Geometry: final body of the model. Coordinates: model frame, mm. A direction names the side the tool comes from. Round coordinates to 2 decimals unless told otherwise and drop trailing zeros. Write each loop counter-clockwise with the first axis right and the second up, starting at its lowest first coordinate (ties: lowest second). Pieces come first, ordered by that corner, then holes. Notation, with made-up numbers: M 33.5,-32 L 83.5,-32 A27 cw 83.5,-12 Z; hole C -1,85 d2. An arc over 180 degrees is marked long. Use one line per item in the form item = value. Start each with the question number.
Item 1: Section query C-C (z = 488.5). Return loops of the section in (x, y), and give its area (3 significant figures).
Item 2: Section query B-B (y = 23). Return loops of the section in (x, z), and give its area (3 significant figures).
Item 3: Pull-direction query (Y, two-part tool) for faces 6 (the flat face through (-216, -876.829, 392)), 7 (the flat face through (-216, 68.051, 807)), 8 (the flat face through (-216, -142, 731.52)), 9 (the flat face through (18.22, 418.85, 450.8)); classes: pulls with the +Y half, pulls with the -Y half, needs draft (parallel to the pull), parting line crosses it, or undercut.
Item 4: Ray query, probe 1 along X at (y, z) = (-590, 610); probe 2 along Y at (x, z) = (31.5, 634.5); probe 3 along X at (y, z) = (-269, 721.5). Return the intervals inside material, ascending.
Item 5: Section query A-A (z = 141). Return loops of the section in (x, y).
Item 6: Pin query (flat end, axial travel): pin 1 Ø15 at (x, z) = (-250.5, 463.5) entering from +Y; pin 2 Ø1.5 at (y, z) = (192, 397.5) entering from -X; pin 3 Ø24.5 at (x, z) = (-218.5, 789) entering from -Y; pin 4 Ø5 at (x, y) = (-175.5, -206) entering from -Z. Return the tip coordinate at first contact, or that it passes through.
Item 7: Section query D-D (x = 8). Return loops of the section in (y, z).
Item 8: Reachability of faces 1 (the flat face through (-216, -450.109, 392)), 2 (the flat face through (-216, -660, 883.92)), 3 (the flat face through (10, -307, 914.4)), 4 (the flat face through (-216, -142, 91.44)), 5 (the flat face through (-216, -876.829, 807)) from +Z, -Z, +X, -X, +Y, -Y: full face, straight path, thin tool, end or side. Return the list, or none.
from build123d import *

# Parameters (mm, degrees)
F1_DEPTH = 914.4
F2_W     = 426.72
F2_H     = 609.6
F2_H_2   = 152.4
F3_DEPTH = 30.48
F4_W     = 15.24
F4_H     = 121.92
F5_DEPTH = 30.48


with BuildPart() as f1:
    # F0 (on Top) → F1 (new body)
    with BuildSketch(Plane.XY):
        Polygon((318.431516, 193.019261), (-290.511489, 651.093946), (-280.741865, 224.485797), (-201.23198, 132.059261), (-201.23198, -934.740739), (318.431516, -934.740739), align=None)
    extrude(amount=F1_DEPTH)

    # F2 (on face) → F3 (join)
    with BuildSketch(Plane(origin=(-201.23198, 0, 0), x_dir=(0, -1, 0), z_dir=(-1, 0, 0))):
        with Locations((145.308739, 396.24)):
            Rectangle(F2_W, F2_H)
        with Locations((663.468739, 396.24)):
            Rectangle(F2_W, F2_H)
        with Locations((145.308739, 807.72)):
            Rectangle(F2_W, F2_H_2)
        with Locations((663.468739, 807.72)):
            Rectangle(F2_W, F2_H_2)
    extrude(amount=F3_DEPTH)

    # F4 (on face) → F5 (join)
    with BuildSketch(Plane(origin=(-231.71198, 0, 0), x_dir=(0, -1, 0), z_dir=(-1, 0, 0))):
        with Locations((329.712739, 470.0016)):
            Rectangle(F4_W, F4_H)
        with Locations((479.064739, 470.0016)):
            Rectangle(F4_W, F4_H)
    extrude(amount=F5_DEPTH)


solid = f1.part
Working result:
q1.outline = M -290.51,651.09 L -280.74,224.49 L -201.23,132.06 L -201.23,68.05 L -231.71,68.05 L -231.71,-322.09 L -262.19,-322.09 L -262.19,-337.33 L -231.71,-337.33 L -231.71,-358.67 L -201.23,-358.67 L -201.23,-450.11 L -231.71,-450.11 L -231.71,-471.44 L -262.19,-471.44 L -262.19,-486.68 L -231.71,-486.68 L -231.71,-876.83 L -201.23,-876.83 L -201.23,-934.74 L 318.43,-934.74 L 318.43,193.02 Z
q1.area = 751,000 mm²
q2.outline = M -231.71,91.44 L -201.23,91.44 L -201.23,0 L 318.43,0 L 318.43,914.4 L -201.23,914.4 L -201.23,883.92 L -231.71,883.92 L -231.71,731.52 L -201.23,731.52 L -201.23,701.04 L -231.71,701.04 Z
q2.area = 498,000 mm²
q3.face_6 = pulls with the -Y half
q3.face_7 = undercut
q3.face_8 = needs draft
q3.face_9 = pulls with the +Y half
q4.probe_1 = -231.71 to 318.43
q4.probe_2 = -934.74 to 408.86
q4.probe_3 = -201.23 to 318.43
q5.outline = M -290.51,651.09 L -280.74,224.49 L -201.23,132.06 L -201.23,68.05 L -231.71,68.05 L -231.71,-358.67 L -201.23,-358.67 L -201.23,-450.11 L -231.71,-450.11 L -231.71,-876.83 L -201.23,-876.83 L -201.23,-934.74 L 318.43,-934.74 L 318.43,193.02 Z
q6.pin_1 = 626.64
q6.pin_2 = -253.44
q6.pin_3 = -876.83
q6.pin_4 = 0
q7.outline = M -934.74,0 L 426.54,0 L 426.54,914.4 L -934.74,914.4 Z
q8.face_1 = +Z, -Z, -X
q8.face_2 = +Z, -X, -Y
q8.face_3 = +Z, +X, -X, +Y, -Y
q8.face_4 = -Z, -X, -Y
q8.face_5 = +Z, -Z, -X, -Y
